Geometry check sheet. Reference: the model listing, model coordinates, mm. Face numbers are marked on the shaded views. A direction names the side the tool comes from. Round coordinates to 2 decimals unless told otherwise and drop trailing zeros. Use a Markdown table: item, result. Add a question column.
(1) Mould release check, pull along X, two halves, no side actions. Record for the marked faces 3, 4 and 5: released by +X, released by -X, zero draft, split by the parting line, or undercut.
(2) Section check A-A on z = 6.25. Give the number of separate pieces and of enclosed holes in the cut face, then the cut area to 3 significant figures.
(3) Gauge pin test, flat ends, axial feed: P1, Ø5, axis at y = 3.5, z = 11, coming from the -X side; P2, Ø5, axis at y = -14, z = 8, coming from the +X side; P3, Ø3, axis at x = 0, y = -14, coming from the -Z side; P4, Ø4, axis at y = 3, z = -0.5, coming from the +X side. Record the tip position at first contact, or that the pin passes through.
(4) Access from +Z, -Z, +X, -X, +Y, -Y to the whole of each face (thin tool, end or side, straight path). Record for the marked faces 1 and 2.
(5) Thickness scan on line 1 along Y through (x, z) = (0, -1.75); line 2 along Y through (x, z) = (0, 2); line 3 along X through (y, z) = (-7, -6.6). Record the ranges inside material, lowest first. Write a range as [from, to].
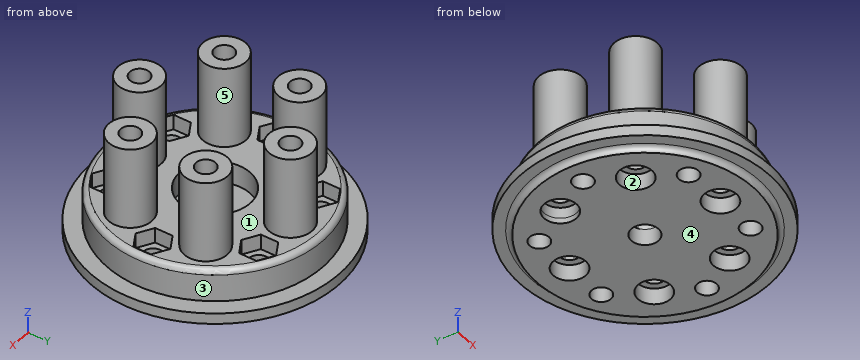
```python
from build123d import *

# Parameters (mm, degrees)
SKETCH_1_R          = 4
EXTRUDE_1_DEPTH     = 20
EXTRUDE_1_2_DEPTH   = 20
EXTRUDE_1_3_DEPTH   = 20
EXTRUDE_1_4_DEPTH   = 20
EXTRUDE_1_5_DEPTH   = 20
EXTRUDE_1_6_DEPTH   = 20
SKETCH_2_R          = 20
EXTRUDE_2_DEPTH     = 6
SKETCH_3_R          = 1.8
CUT_EXTRUDE_1_DEPTH = 39.418745425
SKETCH_4_R          = 6.5
CUT_EXTRUDE_2_DEPTH = 35.641016151
SKETCH_5_R          = 23
SKETCH_5_R_2        = 20
EXTRUDE_3_DEPTH     = 2
CUT_EXTRUDE_START   = -5
SKETCH_7_R          = 4
CUT_EXTRUDE_3_DEPTH = 5
SKETCH_8_R          = 20
SKETCH_8_R_2        = 2.5
SKETCH_8_R_3        = 1.8
EXTRUDE_6_DEPTH     = 4
SKETCH_12_R         = 3
CUT_EXTRUDE_4_DEPTH = 3
CUT_EXTRUDE_5_DEPTH = 2.8
SKETCH_14_R         = 1.8
CUT_EXTRUDE_6_DEPTH = 38.078834933
SKETCH_15_R         = 20
SKETCH_15_R_2       = 2.5
SKETCH_15_R_3       = 3
SKETCH_15_R_4       = 1.8
EXTRUDE_7_DEPTH     = 1
SKETCH_16_R         = 3
SKETCH_16_R_2       = 1.8
EXTRUDE_8_DEPTH     = 1
EXTRUDE_START       = 4
SKETCH_17_R         = 23
SKETCH_17_R_2       = 20
EXTRUDE_9_DEPTH     = 2
CUT_EXTRUDE_START_2 = -2
SKETCH_18_R         = 23
SKETCH_18_R_2       = 20
CUT_EXTRUDE_7_DEPTH = 2
FILLET_3_R          = 1
EXTRUDE_START_2     = 2
SKETCH_19_R         = 6.5
SKETCH_19_R_2       = 2.5
EXTRUDE_10_DEPTH    = 2
SKETCH_21_R         = 20
CUT_EXTRUDE_8_DEPTH = 2
SKETCH_22_R         = 3
CUT_EXTRUDE_9_DEPTH = 2
FILLET_4_R          = 1


with BuildPart() as part:
    # Sketch 1 → Extrude 1 (new body)
    with BuildSketch(Plane.XY):
        with Locations((0, 14)):
            Circle(SKETCH_1_R)
    extrude(amount=EXTRUDE_1_DEPTH)



with BuildPart() as body_2:
    # Sketch 1 → Extrude 1 2 (new body)
    with BuildSketch(Plane.XY):
        with Locations((12.124355653, 7)):
            Circle(SKETCH_1_R)
    extrude(amount=EXTRUDE_1_2_DEPTH)


with BuildPart() as body_3:
    # Sketch 1 → Extrude 1 3 (new body)
    with BuildSketch(Plane.XY):
        with Locations((12.124355653, -7)):
            Circle(SKETCH_1_R)
    extrude(amount=EXTRUDE_1_3_DEPTH)


with BuildPart() as body_4:
    # Sketch 1 → Extrude 1 4 (new body)
    with BuildSketch(Plane.XY):
        with Locations((0, -14)):
            Circle(SKETCH_1_R)
    extrude(amount=EXTRUDE_1_4_DEPTH)


with BuildPart() as body_5:
    # Sketch 1 → Extrude 1 5 (new body)
    with BuildSketch(Plane.XY):
        with Locations((-12.124355653, -7)):
            Circle(SKETCH_1_R)
    extrude(amount=EXTRUDE_1_5_DEPTH)


with BuildPart() as body_6:
    # Sketch 1 → Extrude 1 6 (new body)
    with BuildSketch(Plane.XY):
        with Locations((-12.124355653, 7)):
            Circle(SKETCH_1_R)
    extrude(amount=EXTRUDE_1_6_DEPTH)


with BuildPart() as part_1:
    add(part.part)

    add(body_2.part)  # Extrude 2 merges body 2

    add(body_3.part)  # Extrude 2 merges body 3

    add(body_4.part)  # Extrude 2 merges body 4

    add(body_5.part)  # Extrude 2 merges body 5

    add(body_6.part)  # Extrude 2 merges body 6
    # Sketch 2 → Extrude 2 (add)
    with BuildSketch(Plane(origin=(0, 0, 0), x_dir=(-1, 0, 0), z_dir=(0, 0, -1))):
        Circle(SKETCH_2_R)
    extrude(amount=EXTRUDE_2_DEPTH)

    # Sketch 3 → Cut-Extrude 1 (cut, through all)
    with BuildSketch(Plane.XY.offset(20)):
        with Locations((0, 14)):
            Circle(SKETCH_3_R)
        with Locations((12.124355653, 7)):
            Circle(SKETCH_3_R)
        with Locations((12.124355653, -7)):
            Circle(SKETCH_3_R)
        with Locations((0, -14)):
            Circle(SKETCH_3_R)
        with Locations((-12.124355653, -7)):
            Circle(SKETCH_3_R)
        with Locations((-12.124355653, 7)):
            Circle(SKETCH_3_R)
    extrude(amount=-CUT_EXTRUDE_1_DEPTH, mode=Mode.SUBTRACT)

    # Sketch 4 → Cut-Extrude 2 (cut, through all)
    with BuildSketch(Plane.XY):
        Circle(SKETCH_4_R)
    extrude(amount=-CUT_EXTRUDE_2_DEPTH, mode=Mode.SUBTRACT)

    # Sketch 5 → Extrude 3 (add)
    with BuildSketch(Plane.XY):
        Circle(SKETCH_5_R)
        Circle(SKETCH_5_R_2, mode=Mode.SUBTRACT)
    extrude(amount=-EXTRUDE_3_DEPTH)

    # Sketch 7 → Cut-Extrude 3 (cut)
    with BuildSketch(Plane.XY.offset(20).offset(CUT_EXTRUDE_START)):
        with Locations(Location((0, -14, 0), (0, 0, 180))):
            Circle(SKETCH_7_R)
        with Locations(Location((-12.124355653, -7, 0), (0, 0, 180))):
            Circle(SKETCH_7_R)
        with Locations(Location((-12.124355653, 7, 0), (0, 0, 180))):
            Circle(SKETCH_7_R)
        with Locations((0, 14)):
            Circle(SKETCH_7_R)
        with Locations(Location((12.124355653, 7, 0), (0, 0, 180))):
            Circle(SKETCH_7_R)
        with Locations(Location((12.124355653, -7, 0), (0, 0, 180))):
            Circle(SKETCH_7_R)
    extrude(amount=CUT_EXTRUDE_3_DEPTH, mode=Mode.SUBTRACT)

    # Sketch 8 → Extrude 6 (add)
    with BuildSketch(Plane(origin=(0, 0, -6), x_dir=(-1, 0, 0), z_dir=(0, 0, -1))):
        with Locations(Location((0, 0, 0), (0, 0, 180))):
            Circle(SKETCH_8_R)
        Circle(SKETCH_8_R_2, mode=Mode.SUBTRACT)
        with Locations(Location((12.124355653, 7, 0), (0, 0, 180))):
            Circle(SKETCH_8_R_3, mode=Mode.SUBTRACT)
        with Locations(Location((12.124355653, -7, 0), (0, 0, 180))):
            Circle(SKETCH_8_R_3, mode=Mode.SUBTRACT)
        with Locations(Location((0, -14, 0), (0, 0, 180))):
            Circle(SKETCH_8_R_3, mode=Mode.SUBTRACT)
        with Locations(Location((-12.124355653, -7, 0), (0, 0, 180))):
            Circle(SKETCH_8_R_3, mode=Mode.SUBTRACT)
        with Locations(Location((-12.124355653, 7, 0), (0, 0, 180))):
            Circle(SKETCH_8_R_3, mode=Mode.SUBTRACT)
        with Locations(Location((0, 14, 0), (0, 0, 180))):
            Circle(SKETCH_8_R_3, mode=Mode.SUBTRACT)
    extrude(amount=EXTRUDE_6_DEPTH)

    # Sketch 12 → Cut-Extrude 4 (cut)
    with BuildSketch(Plane(origin=(0, 0, -10), x_dir=(-1, 0, 0), z_dir=(0, 0, -1))):
        with Locations((0, 14)):
            Circle(SKETCH_12_R)
        with Locations((12.124355653, 7)):
            Circle(SKETCH_12_R)
        with Locations((12.124355653, -7)):
            Circle(SKETCH_12_R)
        with Locations((0, -14)):
            Circle(SKETCH_12_R)
        with Locations((-12.124355653, -7)):
            Circle(SKETCH_12_R)
        with Locations((-12.124355653, 7)):
            Circle(SKETCH_12_R)
    extrude(amount=-CUT_EXTRUDE_4_DEPTH, mode=Mode.SUBTRACT)

    # Sketch 13 → Cut-Extrude 5 (cut)
    with BuildSketch(Plane.XY):
        Polygon((16, 3.233161507), (13.2, 1.616580754), (13.2, -1.616580754), (16, -3.233161507), (18.8, -1.616580754), (18.8, 1.616580754), align=None)
        Polygon((10.8, -12.239825707), (8, -10.623244953), (5.2, -12.239825707), (5.2, -15.472987214), (8, -17.089567968), (10.8, -15.472987214), align=None)
        Polygon((-5.2, -15.472987214), (-5.2, -12.239825707), (-8, -10.623244953), (-10.8, -12.239825707), (-10.8, -15.472987214), (-8, -17.089567968), align=None)
        Polygon((-16, -3.233161507), (-13.2, -1.616580754), (-13.2, 1.616580754), (-16, 3.233161507), (-18.8, 1.616580754), (-18.8, -1.616580754), align=None)
        Polygon((-10.8, 12.239825707), (-8, 10.623244953), (-5.2, 12.239825707), (-5.2, 15.472987214), (-8, 17.089567968), (-10.8, 15.472987214), align=None)
        Polygon((5.2, 15.472987214), (5.2, 12.239825707), (8, 10.623244953), (10.8, 12.239825707), (10.8, 15.472987214), (8, 17.089567968), align=None)
    extrude(amount=-CUT_EXTRUDE_5_DEPTH, mode=Mode.SUBTRACT)

    # Sketch 14 → Cut-Extrude 6 (cut, through all)
    with BuildSketch(Plane.XY.offset(-2.8)):
        with Locations((16, 0)):
            Circle(SKETCH_14_R)
        with Locations((8, -13.856406461)):
            Circle(SKETCH_14_R)
        with Locations((-8, -13.856406461)):
            Circle(SKETCH_14_R)
        with Locations((-16, 0)):
            Circle(SKETCH_14_R)
        with Locations((-8, 13.856406461)):
            Circle(SKETCH_14_R)
        with Locations((8, 13.856406461)):
            Circle(SKETCH_14_R)
    extrude(amount=-CUT_EXTRUDE_6_DEPTH, mode=Mode.SUBTRACT)

    # Sketch 15 → Extrude 7 (add)
    with BuildSketch(Plane(origin=(0, 0, -10), x_dir=(-1, 0, 0), z_dir=(0, 0, -1))):
        with Locations(Location((0, 0, 0), (0, 0, 180))):
            Circle(SKETCH_15_R)
        Circle(SKETCH_15_R_2, mode=Mode.SUBTRACT)
        with Locations((0, 14)):
            Circle(SKETCH_15_R_3, mode=Mode.SUBTRACT)
        with Locations(Location((-8, 13.856406461, 0), (0, 0, 180))):
            Circle(SKETCH_15_R_4, mode=Mode.SUBTRACT)
        with Locations(Location((8, 13.856406461, 0), (0, 0, 180))):
            Circle(SKETCH_15_R_4, mode=Mode.SUBTRACT)
        with Locations(Location((16, 0, 0), (0, 0, 180))):
            Circle(SKETCH_15_R_4, mode=Mode.SUBTRACT)
        with Locations(Location((8, -13.856406461, 0), (0, 0, 180))):
            Circle(SKETCH_15_R_4, mode=Mode.SUBTRACT)
        with Locations(Location((-8, -13.856406461, 0), (0, 0, 180))):
            Circle(SKETCH_15_R_4, mode=Mode.SUBTRACT)
        with Locations(Location((-16, 0, 0), (0, 0, 180))):
            Circle(SKETCH_15_R_4, mode=Mode.SUBTRACT)
        with Locations((12.124355653, 7)):
            Circle(SKETCH_15_R_3, mode=Mode.SUBTRACT)
        with Locations((12.124355653, -7)):
            Circle(SKETCH_15_R_3, mode=Mode.SUBTRACT)
        with Locations((0, -14)):
            Circle(SKETCH_15_R_3, mode=Mode.SUBTRACT)
        with Locations((-12.124355653, -7)):
            Circle(SKETCH_15_R_3, mode=Mode.SUBTRACT)
        with Locations((-12.124355653, 7)):
            Circle(SKETCH_15_R_3, mode=Mode.SUBTRACT)
    extrude(amount=EXTRUDE_7_DEPTH)

    # Sketch 16 → Extrude 8 (add)
    # profile 1 of 6: a face of its own
    with BuildSketch(Plane(origin=(0, 0, -7), x_dir=(-1, 0, 0), z_dir=(0, 0, -1))):
        with Locations((0, -14)):
            Circle(SKETCH_16_R)
        with Locations(Location((0, -14, 0), (0, 0, 180))):
            Circle(SKETCH_16_R_2, mode=Mode.SUBTRACT)
    # profile 2 of 6: a face of its own
    with BuildSketch(Plane(origin=(0, 0, -7), x_dir=(-1, 0, 0), z_dir=(0, 0, -1))):
        with Locations((-12.124355653, -7)):
            Circle(SKETCH_16_R)
        with Locations(Location((-12.124355653, -7, 0), (0, 0, 180))):
            Circle(SKETCH_16_R_2, mode=Mode.SUBTRACT)
    # profile 3 of 6: a face of its own
    with BuildSketch(Plane(origin=(0, 0, -7), x_dir=(-1, 0, 0), z_dir=(0, 0, -1))):
        with Locations((-12.124355653, 7)):
            Circle(SKETCH_16_R)
        with Locations(Location((-12.124355653, 7, 0), (0, 0, 180))):
            Circle(SKETCH_16_R_2, mode=Mode.SUBTRACT)
    # profile 4 of 6: a face of its own
    with BuildSketch(Plane(origin=(0, 0, -7), x_dir=(-1, 0, 0), z_dir=(0, 0, -1))):
        with Locations((0, 14)):
            Circle(SKETCH_16_R)
        with Locations(Location((0, 14, 0), (0, 0, 180))):
            Circle(SKETCH_16_R_2, mode=Mode.SUBTRACT)
    # profile 5 of 6: a face of its own
    with BuildSketch(Plane(origin=(0, 0, -7), x_dir=(-1, 0, 0), z_dir=(0, 0, -1))):
        with Locations((12.124355653, 7)):
            Circle(SKETCH_16_R)
        with Locations(Location((12.124355653, 7, 0), (0, 0, 180))):
            Circle(SKETCH_16_R_2, mode=Mode.SUBTRACT)
    # profile 6 of 6: a face of its own
    with BuildSketch(Plane(origin=(0, 0, -7), x_dir=(-1, 0, 0), z_dir=(0, 0, -1))):
        with Locations((12.124355653, -7)):
            Circle(SKETCH_16_R)
        with Locations(Location((12.124355653, -7, 0), (0, 0, 180))):
            Circle(SKETCH_16_R_2, mode=Mode.SUBTRACT)
    extrude(amount=EXTRUDE_8_DEPTH)

    # Sketch 17 → Extrude 9 (add)
    with BuildSketch(Plane(origin=(0, 0, -2), x_dir=(-1, 0, 0), z_dir=(0, 0, -1)).offset(EXTRUDE_START)):
        with Locations(Location((0, 0, 0), (0, 0, 180))):
            Circle(SKETCH_17_R)
        with Locations(Location((0, 0, 0), (0, 0, 180))):
            Circle(SKETCH_17_R_2, mode=Mode.SUBTRACT)
    extrude(amount=EXTRUDE_9_DEPTH)

    # Sketch 18 → Cut-Extrude 7 (cut)
    with BuildSketch(Plane(origin=(0, 0, -2), x_dir=(-1, 0, 0), z_dir=(0, 0, -1)).offset(CUT_EXTRUDE_START_2)):
        Circle(SKETCH_18_R)
        Circle(SKETCH_18_R_2, mode=Mode.SUBTRACT)
    extrude(amount=CUT_EXTRUDE_7_DEPTH, mode=Mode.SUBTRACT)

    # Fillet 3
    fillet_3_edges = [part_1.edges().sort_by_distance(p)[0] for p in [
        (20, 0, 0),
    ]]
    fillet(fillet_3_edges, radius=FILLET_3_R)

    # Sketch 19 → Extrude 10 (add)
    with BuildSketch(Plane.XY.offset(-6).offset(EXTRUDE_START_2)):
        Circle(SKETCH_19_R)
        Circle(SKETCH_19_R_2, mode=Mode.SUBTRACT)
    extrude(amount=-EXTRUDE_10_DEPTH)

    # Sketch 21 → Cut-Extrude 8 (cut)
    with BuildSketch(Plane(origin=(0, 0, -11), x_dir=(-1, 0, 0), z_dir=(0, 0, -1)).offset(CUT_EXTRUDE_START_2)):
        Circle(SKETCH_21_R)
    extrude(amount=CUT_EXTRUDE_8_DEPTH, mode=Mode.SUBTRACT)

    # Sketch 22 → Cut-Extrude 9 (cut)
    with BuildSketch(Plane(origin=(0, 0, -8), x_dir=(-1, 0, 0), z_dir=(0, 0, -1)).offset(CUT_EXTRUDE_START_2)):
        with Locations((0, 14)):
            Circle(SKETCH_22_R)
        with Locations((-12.124355653, 7)):
            Circle(SKETCH_22_R)
        with Locations((12.124355653, 7)):
            Circle(SKETCH_22_R)
        with Locations((12.124355653, -7)):
            Circle(SKETCH_22_R)
        with Locations((0, -14)):
            Circle(SKETCH_22_R)
        with Locations((-12.124355653, -7)):
            Circle(SKETCH_22_R)
    extrude(amount=CUT_EXTRUDE_9_DEPTH, mode=Mode.SUBTRACT)

    # Fillet 4
    fillet_4_edges = [part_1.edges().sort_by_distance(p)[0] for p in [
        (-20, 0, -8),
    ]]
    fillet(fillet_4_edges, radius=FILLET_4_R - 0.0001)  # a hair under: the kernel refuses the full size


solid = part_1.part
```
Check sheet entries:
| question | item | result |
|---|---|---|
| 1 | face 3 | split by the parting line |
| 1 | face 4 | zero draft |
| 1 | face 5 | undercut |
| 2 | separate pieces | 6 |
| 2 | enclosed holes | 6 |
| 2 | area | 241 mm2 |
| 3 | P1 | stops at x = -16 |
| 3 | P2 | stops at x = 4 |
| 3 | P3 | passes through |
| 3 | P4 | stops at x = 19.97 |
| 4 | face 1 | +Z |
| 4 | face 2 | -Z |
| 5 | line 1 | y = [-20, -15.8], [-12.2, -6.5], [6.5, 12.2], [15.8, 20] |
| 5 | line 2 | y = [-18, -15.8], [-12.2, -10], [10, 12.2], [15.8, 18] |
| 5 | line 3 | x = [-21.91, -15.12], [-9.12, 9.12], [15.12, 21.91] |
